Geometry: final body of the model. Coordinates: model frame, mm. A direction names the side the tool comes from. Give positions to 0.01 mm unless a question says otherwise; leave off trailing zeros. Loops run counter-clockwise (first coordinate to the right, second up) from the corner with the lowest first, then second, coordinate; pieces in that order, holes last.
from build123d import *

# Parameters (mm, degrees)
SKETCH1_R           = 40
SKETCH1_R_2         = 39
BOSS_EXTRUDE1_DEPTH = 193
CUT_EXTRUDE3_START  = -80
CUT_EXTRUDE3_DEPTH  = 150
CUT_EXTRUDE4_DEPTH  = 35
SKETCH22_R          = 1.7
CUT_EXTRUDE5_DEPTH  = 5.3
CIRPATTERN1_COUNT   = 4
SKETCH24_W          = 31.232190918
SKETCH24_H          = 10.655653456
CUT_EXTRUDE6_DEPTH  = 13.3


with BuildPart() as part:
    # Sketch1 → Boss-Extrude1 (new body)
    with BuildSketch(Plane(origin=(0, 63, 0), x_dir=(1, 0, 0), z_dir=(0, 1, 0))):
        with Locations(Location((0, 0, 0), (0, 0, 270))):
            Circle(SKETCH1_R)
        with Locations(Location((0, 0, 0), (0, 0, 270))):
            Circle(SKETCH1_R_2, mode=Mode.SUBTRACT)
    extrude(amount=BOSS_EXTRUDE1_DEPTH)

    # Sketch11 → Cut-Extrude3 (cut)
    with BuildSketch(Plane(origin=(0, 256, 0), x_dir=(1, 0, 0), z_dir=(0, 1, 0)).offset(CUT_EXTRUDE3_START)):
        Polygon((16.455199497, 17.541777329), (2.860582691, 23.881051254), (12.76219936, 45.115136729), (26.356816166, 38.775862804), align=None)
        Polygon((-17.541777329, 16.455199497), (-23.881051254, 2.860582691), (-45.115136729, 12.76219936), (-38.775862804, 26.356816166), align=None)
        Polygon((17.541777329, -16.455199497), (23.881051254, -2.860582691), (45.115136729, -12.76219936), (38.775862804, -26.356816166), align=None)
        Polygon((-16.455199497, -17.541777329), (-2.860582691, -23.881051254), (-12.76219936, -45.115136729), (-26.356816166, -38.775862804), align=None)
        Polygon((-43.620574428, -12.065273515), (-21.566495936, -1.781287822), (-15.22722201, -15.375904627), (-37.281300502, -25.659890321), align=None)
        Polygon((-12.065273515, 43.620574428), (-1.781287822, 21.566495936), (-15.375904627, 15.22722201), (-25.659890321, 37.281300502), align=None)
        Polygon((43.620574428, 12.065273515), (21.566495936, 1.781287822), (15.22722201, 15.375904627), (37.281300502, 25.659890321), align=None)
        Polygon((12.065273515, -43.620574428), (1.781287822, -21.566495936), (15.375904627, -15.22722201), (25.659890321, -37.281300502), align=None)
    extrude(amount=-CUT_EXTRUDE3_DEPTH, mode=Mode.SUBTRACT)

    # Sketch20 → Cut-Extrude4 (cut)
    with BuildSketch(Plane(origin=(30.542754268, 0, -30.542754268), x_dir=(-0.7043828553421385, 0.08769028567936554, -0.7043828553404231), z_dir=(0.7071067811856864, -4.163336342344337e-15, -0.7071067811874089))):
        with BuildLine():
            Line((7.051429642, 237.476570021), (5.590509483, 220.880747887))
            ThreePointArc((5.590509483, 220.880747887), (6.847288676, 216.88728279), (10.559772016, 214.952153629))
            Line((10.559772016, 214.952153629), (27.155594149, 213.491233469))
            ThreePointArc((27.155594149, 213.491233469), (31.149059247, 214.748012662), (33.084188408, 218.460496002))
            Line((33.084188408, 218.460496002), (34.545108567, 235.056318136))
            ThreePointArc((34.545108567, 235.056318136), (33.288329374, 239.049783233), (29.575846034, 240.984912394))
            Line((29.575846034, 240.984912394), (12.980023901, 242.445832553))
            ThreePointArc((12.980023901, 242.445832553), (8.986558804, 241.189053361), (7.051429642, 237.476570021))
        make_face()
    extrude(amount=-CUT_EXTRUDE4_DEPTH, mode=Mode.SUBTRACT)

    # Sketch22 → Cut-Extrude5 (cut)
    with BuildSketch(Plane(origin=(24.169183991, 0, -24.169183991), x_dir=(0.7071067811865483, 0, 0.7071067811865468), z_dir=(-0.7071067811865468, 0, 0.7071067811865483))):
        with Locations((0, 68)):
            Circle(SKETCH22_R)
    cut_extrude5 = extrude(amount=-CUT_EXTRUDE5_DEPTH, mode=Mode.SUBTRACT)

    # CirPattern1: Cut-Extrude5 ×4 about axis
    cirpattern1_axis = Axis((0, 0, 0), (0, 1, 0))
    for i in range(1, CIRPATTERN1_COUNT):
        add(cut_extrude5.rotate(cirpattern1_axis, i * 360 / CIRPATTERN1_COUNT), mode=Mode.SUBTRACT)

    # Sketch24 → Cut-Extrude6 (cut)
    with BuildSketch(Plane(origin=(-28.056295298, 0, 20.384091712), x_dir=(-0.5877852522931263, 0, -0.8090169943744729), z_dir=(0.8090169943744729, 0, -0.5877852522931263))):
        with Locations((3.911568973, 188.130853463)):
            Rectangle(SKETCH24_W, SKETCH24_H)
    extrude(amount=-CUT_EXTRUDE6_DEPTH, mode=Mode.SUBTRACT)


solid = part.part
Item 1: Section query A-A on z = 0. Return loops of the section in (x, y), plus the area to 3 significant figures.
Values follow:
outline: (-40, 63) - (-39, 63) - (-39, 256) - (-40, 256) - close; (39, 63) - (40, 63) - (40, 256) - (39, 256) - close
area: 386 mm2
Item 2: Pin query (flat end, axial travel): pin 1 (2 mm diameter, centred on x = 5, y = 184, fed in from -Z); pin 2 (3.5 mm diameter, centred on x = -35.5, z = 15.5, fed in from -Y); pin 3 (1.5 mm diameter, centred on x = 3.5, y = 222, fed in from -Z). Return the tip coordinate at first contact, or that it passes through.
Values follow:
pin 1: stops at z = -39.8
pin 2: stops at y = 176
pin 3: stops at z = -39.91
Item 3: Section query B-B on x = 0. Return loops of the section in (y, z), plus the area to 3 significant figures.
Values follow:
outline: (63, -40) - (256, -40) - (256, -39) - (63, -39) - close; (63, 39) - (256, 39) - (256, 40) - (63, 40) - close
area: 386 mm2
Item 4: Section query D-D on z = 13.5. Return loops of the section in (x, y), plus the area to 3 significant figures.
Values follow:
outline: (-37.65, 176) - (-36.59, 176) - (-36.59, 182.8) - (-37.65, 182.8) - close; (-37.65, 193.46) - (-36.59, 193.46) - (-36.59, 256) - (-37.65, 256) - close; (36.59, 176) - (37.65, 176) - (37.65, 256) - (36.59, 256) - close
area: 159 mm2
Item 5: Draft query along Y for faces 3 (the face through (28, 242.65, -28)), 4 (the face through (36, 176, 16)), 5 (the face through (-38.3, 256, 8.7)), 6 (the face through (17.879, 241.005, -35.189)). Return one class per face: +Y half, -Y half, draft (parallel to the pull), parting line (faces both ways), or undercut.
Values follow:
face 3: undercut
face 4: -Y half
face 5: +Y half
face 6: undercut
Item 6: Section query C-C on y = 94. Give the number of separate pieces and of enclosed holes in the cut face, plus the area to 3 significant figures.
Values follow:
separate pieces: 8
enclosed holes: 0
area: 127 mm2
Item 7: Set-up query: faces 1 (the face through (28, 63, -28)), 2 (the face through (28, 215.05, -28)). Return all of +Z, -Z, +X, -X, +Y, -Y with unobstructed straight access to the full face (end or side cutting, diameter ignored); none if empty.
Values follow:
face 1: +Z, -Z, +X, -X, -Y
face 2: -Z, +X
Item 8: Ray query, probe 1 along X at (y, z) = (184, 0); probe 2 along X at (y, z) = (220.5, 36). Return the intervals inside material, ascending.
Values follow:
probe 1: x = -40 to -39, 39 to 40
probe 2: x = -17.44 to -15, 15 to 17.44
